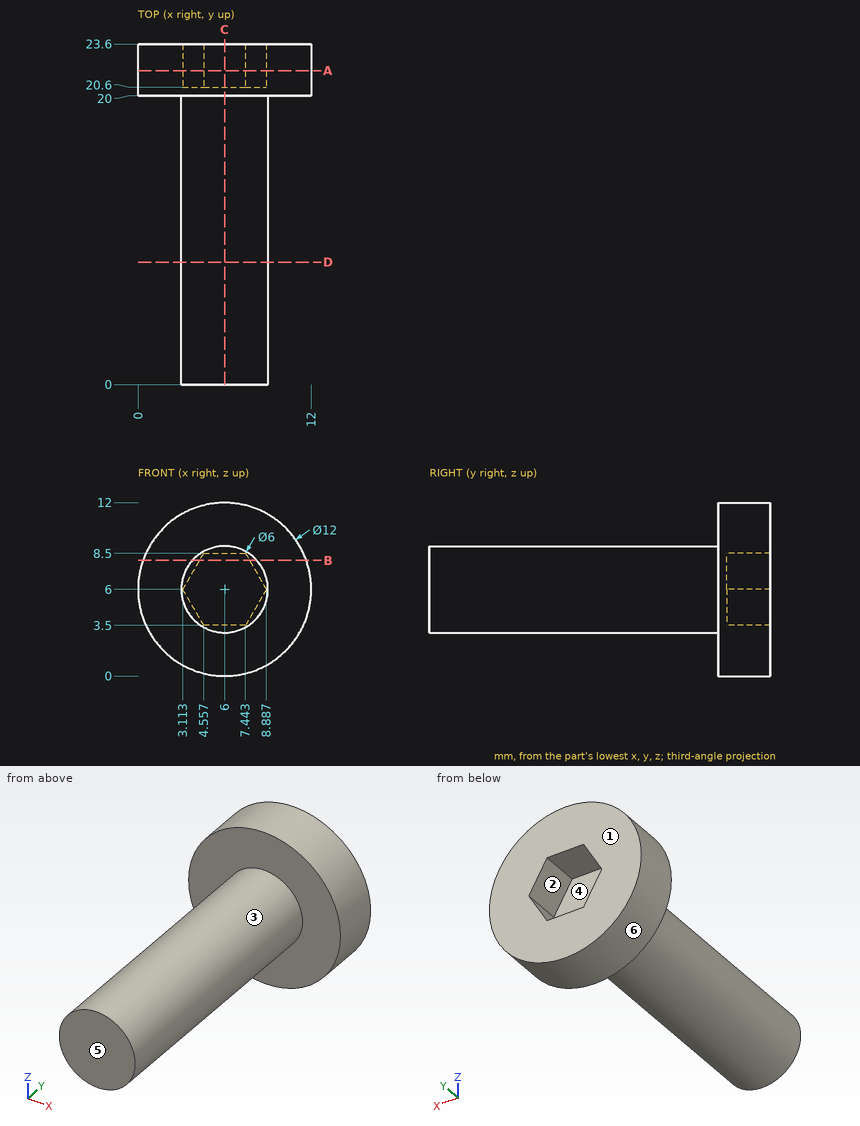
The drawing under review shows one solid part. Ordinate dimensions are in mm from its lowest x, y, z. A direction names the side the tool comes from. Round coordinates to 2 decimals unless told otherwise and drop trailing zeros. Write each loop counter-clockwise with the first axis right and the second up, starting at its lowest first coordinate (ties: lowest second). Pieces come first, ordered by that corner, then holes.
(1) We need section D-D on y = 8.5. Give the boundary of the cut face in (x, z).
(2) Wall thickness on L1, parallel to Y at x = 11.75, z = 6.5; L2, parallel to Y at x = 4, z = 6.25; L3, parallel to Z at x = 3.25, y = 1.25 (1 decimal): over which ranges is each line inside the solid? List them lowest first.
(3) We need section C-C on x = 6. Give the boundary of the cut face in (y, z), and give its area (3 significant figures).
(4) Mouldability with a two-part tool opening along Z and no side actions: class the marked faces 4, 5 and 6 as +Z half, -Z half, draft (parallel to the pull), parting line (faces both ways), or undercut.
(5) Machinability: for the marked faces 1, 2 and 3, which of the approach directions +Z, -Z, +X, -X, +Y, -Y give a long, thin tool a straight path to every point of the face, cutting with its end or side? Answer none if there is none.
(6) We need section A-A on y = 21.75. Give the boundary of the cut face in (x, z).
(7) Insertion check: pin 1 (6 mm diameter, centred on y = 9, z = 6, fed in from -X); pin 2 (4 mm diameter, centred on x = 3, y = 21, fed in from -Z); pin 3 (1.5 mm diameter, centred on x = 9, y = 20, fed in from +Z); pin 4 (1.5 mm diameter, centred on y = 15, z = 1.5, fed in from +X). Each pin has a flat end and moves straight along its axis. Give the tip position at first contact, or say it passes through.
(8) We need section B-B on z = 8. Give the boundary of the cut face in (x, y).
Findings below:
1. outline: circle Ø6 at (6, 6)
2. L1: y = 20 to 23.6
2. L2: y = 0 to 20.6
2. L3: z = 4.8 to 7.2
3. outline: (0, 3) - (20, 3) - (20, 0) - (23.6, 0) - (23.6, 3.5) - (20.6, 3.5) - (20.6, 8.5) - (23.6, 8.5) - (23.6, 12) - (20, 12) - (20, 9) - (0, 9) - close
3. area: 148 mm2
4. face 4: undercut
4. face 5: draft
4. face 6: parting line
5. face 1: +Z, -Z, +X, -X, +Y
5. face 2: +Y
5. face 3: -Y
6. outline: circle Ø12 at (6, 6); hole (3.11, 6) - (4.56, 3.5) - (7.44, 3.5) - (8.89, 6) - (7.44, 8.5) - (4.56, 8.5) - close
7. pin 1: stops at x = 3
7. pin 2: stops at z = 0.08
7. pin 3: stops at z = 11.56
7. pin 4: passes through
8. outline: (0.34, 20) - (3.76, 20) - (3.76, 0) - (8.24, 0) - (8.24, 20) - (11.66, 20) - (11.66, 23.6) - (7.73, 23.6) - (7.73, 20.6) - (4.27, 20.6) - (4.27, 23.6) - (0.34, 23.6) - close
